Solid Edge part; units mm, degrees
sketch "Sketch1" plane through (0, 0, 0) normal (0, 0, 1) x (1, 0, 0)
  line L0 (43, 0) -> (43, 189)
  line L1 (43, 189) -> (0, 189)
  line L2 (0, 189) -> (0, 0)
  line L3 (0, 0) -> (43, 0)
extrude "Protrusion1" add sketch "Sketch1" along normal blind 1.6
hole "Hole_1" at (4.5, 76.1, 1.6) direction (0, 0, -1) diameter 3.5 end through all
hole "Hole1" at (38.5, 76.1, 1.6) direction (0, 0, -1) diameter 3.5 end through all
hole "Hole2" at (21.5, 6, 1.6) direction (0, 0, -1) diameter 3.5 end through all
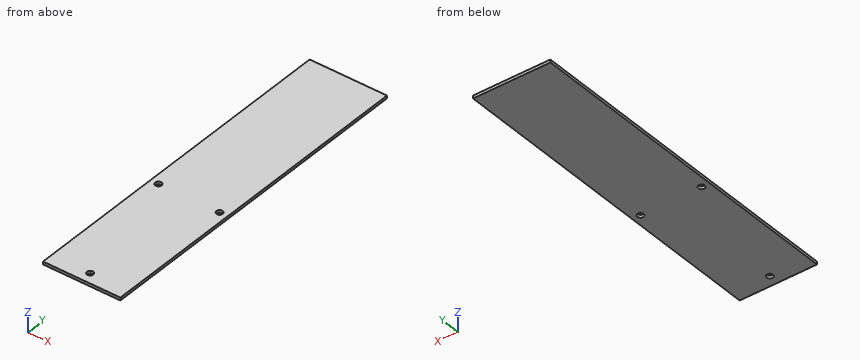
CAD build for the part. Positions are in the model's coordinates, mm. Coordinates: 2 decimals unless noted, no trailing zeros. Write each loop counter-clockwise with the first axis right and the second up, starting at its lowest first coordinate (ties: lowest second). Pieces come first, ordered by that corner, then holes. Notation, with made-up numbers: M 50.5,-7.75 L 58.5,-7.75 A25 cw 58.5,26.25 Z; hole C 22,69.25 d6. An arc over 180 degrees is marked long. Return JSON: item names as keys, results as strings.
Item 1: Slice it at B-B, the plane y = 6. Write the cut outline in (x, z).
Findings below:
{"outline": "M 0,0 L 19.75,0 L 19.75,1.6 L 0,1.6 Z; M 23.25,0 L 43,0 L 43,1.6 L 23.25,1.6 Z"}
Item 2: Slice it at C-C, the plane x = 38.5. Write the cut outline in (y, z), and give its area (3 significant figures).
Findings below:
{"outline": "M 0,0 L 74.35,0 L 74.35,1.6 L 0,1.6 Z; M 77.85,0 L 189,0 L 189,1.6 L 77.85,1.6 Z", "area": "297 mm2"}
Item 3: Slice it at A-A, the plane y = 76.1. Write the cut outline in (x, z), and give its area (3 significant figures).
Findings below:
{"outline": "M 0,0 L 2.75,0 L 2.75,1.6 L 0,1.6 Z; M 6.25,0 L 36.75,0 L 36.75,1.6 L 6.25,1.6 Z; M 40.25,0 L 43,0 L 43,1.6 L 40.25,1.6 Z", "area": "57.6 mm2"}
Item 4: Drop flat-ended pins along their axis: pin 1 Ø4.5 at (x, y) = (21.5, 6) entering from +Z; pin 2 Ø2 at (x, y) = (4.5, 76.1) entering from +Z. Give the stop position or say it passes through.
Findings below:
{"pin 1": "stops at z = 1.6", "pin 2": "passes through"}
Item 5: Probe line 1 (X direction, y = 76.1, z = 0.5); line 2 (Y direction, x = 4.5, z = 0.5); line 3 (X direction, y = 6, z = 0.4). List the from-to ranges inside material, lowest first. Write a range as from..to.
Findings below:
{"line 1": "x = 0..2.75, 6.25..36.75, 40.25..43", "line 2": "y = 0..74.35, 77.85..189", "line 3": "x = 0..19.75, 23.25..43"}
